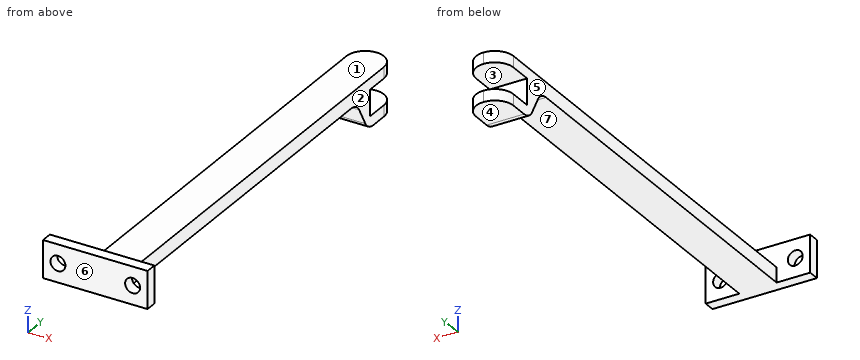
Autodesk Inventor part; units mm, degrees
ref_plane "Work Plane1" through (0, 0, 0) normal (0, 0, 1) x (1, 0, 0)
ref_plane "YZ Plane" through (0, 0, 0) normal (1, 0, 0) x (0, 1, 0)
ref_plane "XZ Plane" through (0, 0, 0) normal (0, 1, 0) x (-1, 0, 0)
sketch "Sketch5" plane through (0, 0, 0) normal (1, 0, 0) x (0, 1, 0)
  line L0 (0, 0) -> (98.4806, 0)
  line L1 (98.4806, 0) -> (98.4806, -3)
  line L2 (98.4806, -3) -> (87.4806, -3)
  line L3 (87.4806, -3) -> (87.4806, -10)
  line L4 (87.4806, -10) -> (98.4806, -10)
  line L5 (98.4806, -10) -> (98.4806, -13)
  line L6 (98.4806, -13) -> (86.4806, -13)
  line L7 (86.4806, -13) -> (81.4806, -4)
  line L8 (-22.5194, 0) -> (0, 0)
  line L9 (-22.5194, -4) -> (81.4806, -4)
  line L10 (-22.5194, -4) -> (-22.5194, 0)
  dimension "d29" = 3
  dimension "d30" = 7
  dimension "d31" = 3
  dimension "d33" = 11
  dimension "d40" = 4
  dimension "d41" = 5
  dimension "d48" = 12
  dimension "d53" = 121
ref_plane "Work Plane1" through (0, 0, 0) normal (0, 0, 1) x (1, 0, 0)
extrude "Extrusion5" add sketch "Sketch5" along normal blind 10
fillet "Fillet1" radius 5 4 edges at (10, 98.4806, -11.5) (0, 98.4806, -11.5) (0, 98.4806, -1.5) (10, 98.4806, -1.5)
fillet "Fillet2" radius 4 2 edges at (5, 86.4806, -13) (5, 81.4806, -4)
sketch "Sketch7" plane through (0, -22.5194, -4) normal (0, 0, -1) x (1, 0, 0)
  line L0 (-9, 0) -> (19, 0)
  line L1 (19, 0) -> (19, 3)
  line L2 (19, 3) -> (-9, 3)
  line L3 (-9, 3) -> (-9, 0)
  line L4 (10, -107.857) -> (0, -107.857)
  line L5 (10, -101.6464) -> (0, -101.6464)
  line L6 (10, 0) -> (10, -101.6464)
  line L7 (0, 0) -> (10, 0)
  line L8 (0, 0) -> (0, -101.6464)
  point P0 (5, 3)
  point P1 (5, -107.857)
  point P2 (5, 0)
  dimension "d58" = 28
  dimension "d59" = 3
extrude "Extrusion6" add sketch "Sketch7" against normal blind 10 contours L3 L2 L1 L0
sketch "Sketch8" plane through (-9, -22.5194, -4) normal (0, 1, 0) x (1, 0, 0)
  line L0 (0, 0) -> (0, -10)
  line L1 (28, 0) -> (28, -10)
  point P0 (9, -4)
  point P1 (4, -5)
  point P2 (24, -5)
  point P3 (0, -5)
  point P4 (28, -5)
  dimension "d69" = 4
  dimension "d70" = 4
hole "Hole3" at (-5, -22.5194, 1) at (15, -22.5194, 1) direction (0, -1, 0) diameter 4 end through all
equation "\"d31\" = d29"
properties part number "2052"
Input: part model. Units: mm. Frame: model coordinates. Face numbers are marked on the shaded views. A direction names the side the tool comes from. Round coordinates to 2 decimals unless told otherwise and drop trailing zeros. Loops run counter-clockwise (first coordinate to the right, second up) from the corner with the lowest first, then second, coordinate; pieces in that order, holes last. Notation, with made-up numbers: (36, -20) -> (82, -20) arc R16 ccw to (82, -9) -> close; hole circle Ø1 at (50.5, 36.25). An arc over 180 degrees is marked (long way). Answer as a JSON object with one key per item and string values. Group by question number.
1) Reachability of the marked faces 5, 6 and 7 from +Z, -Z, +X, -X, +Y, -Y: full face, straight path, thin tool, end or side. Return the list, or none.
2) Ray query, L1, parallel to X at y = -23.8, z = 1; L2, parallel to Z at x = -5, y = -24.45; L3, parallel to X at y = 66, z = -3.25. Return the intervals inside material, ascending.
3) Section query B-B on y = 38.5. Output: boundary loops of the cut face in (x, z), plus the area to 3 significant figures.
4) Section query C-C on z = -7.5. Output: boundary loops of the cut face in (x, y).
5) Pin query (flat end, axial travel): pin 1 (8.5 mm diameter, centred on x = 11, y = 50.5, fed in from -Z); pin 2 (8 mm diameter, centred on x = 4.5, y = 47, fed in from +Z); pin 3 (7.5 mm diameter, centred on x = 7.5, z = -6, fed in from +Y). Return the tip coordinate at first contact, or that it passes through.
6) Section query A-A on x = -5. Output: boundary loops of the cut face in (y, z).
7) Draft query along Z for the marked faces 1, 2, 3 and 4. Return one class per face: +Z half, -Z half, draft (parallel to the pull), parting line (faces both ways), or undercut.
Reply:
{
 "1": {"face 5": "+Z, -Z, -X, +Y", "face 6": "+Z, -Z, +X, -X, -Y", "face 7": "-Z, +X, -X, -Y"},
 "2": {"L1": "x = -9 to -7, -3 to 13, 17 to 19", "L2": "z = -4 to -1, 3 to 6", "L3": "x = 0 to 10"},
 "3": {"outline": "(0, -4) -> (10, -4) -> (10, 0) -> (0, 0) -> close", "area": "40.0 mm2"},
 "4": {"outline": "(0, 83.43) -> (10, 83.43) -> (10, 87.48) -> (0, 87.48) -> close"},
 "5": {"pin 1": "stops at z = -4", "pin 2": "stops at z = 0", "pin 3": "stops at y = 98.47"},
 "6": {"outline": "(-25.52, -4) -> (-22.52, -4) -> (-22.52, -1) -> (-25.52, -1) -> close; (-25.52, 3) -> (-22.52, 3) -> (-22.52, 6) -> (-25.52, 6) -> close"},
 "7": {"face 1": "+Z half", "face 2": "draft", "face 3": "undercut", "face 4": "-Z half"}
}
